```python
from build123d import *

# Parameters (mm, degrees)
EXTRUDE_1_DEPTH      = 0.4
EXTRUDE_2_DEPTH      = 0.6
EXTRUDE_3_DEPTH      = 1.3
EXTRUDE_4_DEPTH      = 1.19
FILLET_1_R           = 0.1
FILLET_2_R           = 0.1
FILLET_3_R           = 0.2
EXTRUDE_5_DEPTH      = 3.5
EXTRUDE_5_DEPTH_BACK = 3.5
EXTRUDE_5_START      = -8.2
SKETCH_3_W           = 10
SKETCH_3_H           = 10
CUT_EXTRUDE_1_DEPTH  = 0.01


with BuildPart() as part:
    # 草图1 → 凸台-拉伸1 (new body)
    with BuildSketch(Plane(origin=(0, 0, 0), x_dir=(1, 0, 0), z_dir=(0, 1, 0))):
        with BuildLine():
            Line((7.3, -8.2), (-7.3, -8.2))
            ThreePointArc((-7.3, -8.2), (-8.007106781, -7.907106781), (-8.3, -7.2))
            Line((-8.3, -7.2), (-8.3, 7.2))
            ThreePointArc((-8.3, 7.2), (-8.007106781, 7.907106781), (-7.3, 8.2))
            Line((-7.3, 8.2), (7.3, 8.2))
            ThreePointArc((7.3, 8.2), (8.007106781, 7.907106781), (8.3, 7.2))
            Line((8.3, 7.2), (8.3, -7.2))
            ThreePointArc((8.3, -7.2), (8.007106781, -7.907106781), (7.3, -8.2))
        make_face()
        with BuildLine():
            Line((7.75, -4.202947793), (7.75, 4.3))
            ThreePointArc((7.75, 4.3), (6.798097039, 6.598097039), (4.5, 7.55))
            ThreePointArc((4.5, 7.55), (4.287867966, 7.637867966), (4.2, 7.85))
            Line((4.2, 7.85), (-4.3, 7.85))
            ThreePointArc((-4.3, 7.85), (-4.387867966, 7.637867966), (-4.6, 7.55))
            ThreePointArc((-4.6, 7.55), (-6.898097039, 6.598097039), (-7.85, 4.3))
            Line((-7.85, 4.3), (-7.85, -4.2))
            ThreePointArc((-7.85, -4.2), (-6.898094676, -6.498099402), (-4.599993316, -7.45))
            ThreePointArc((-4.599993316, -7.45), (-4.387860883, -7.537867748), (-4.299992699, -7.75))
            Line((-4.299992699, -7.75), (4.200007301, -7.75))
            ThreePointArc((4.200007301, -7.75), (4.288905774, -7.539775891), (4.499993425, -7.452947793))
            ThreePointArc((4.499993425, -7.452947793), (6.798094714, -6.501047157), (7.75, -4.202947793))
        make_face(mode=Mode.SUBTRACT)
    extrude(amount=EXTRUDE_1_DEPTH)

    # 草图1<3> → 凸台-拉伸2 (add)
    with BuildSketch(Plane(origin=(0, 0, 0), x_dir=(1, 0, 0), z_dir=(0, 1, 0))):
        with BuildLine():
            Line((7.75, -4.202947793), (7.75, 4.3))
            ThreePointArc((7.75, 4.3), (6.798097039, 6.598097039), (4.5, 7.55))
            ThreePointArc((4.5, 7.55), (4.287867966, 7.637867966), (4.2, 7.85))
            Line((4.2, 7.85), (-4.3, 7.85))
            ThreePointArc((-4.3, 7.85), (-4.387867966, 7.637867966), (-4.6, 7.55))
            ThreePointArc((-4.6, 7.55), (-6.898097039, 6.598097039), (-7.85, 4.3))
            Line((-7.85, 4.3), (-7.85, -4.2))
            ThreePointArc((-7.85, -4.2), (-6.898094676, -6.498099402), (-4.599993316, -7.45))
            ThreePointArc((-4.599993316, -7.45), (-4.387860883, -7.537867748), (-4.299992699, -7.75))
            Line((-4.299992699, -7.75), (4.200007301, -7.75))
            ThreePointArc((4.200007301, -7.75), (4.288905774, -7.539775891), (4.499993425, -7.452947793))
            ThreePointArc((4.499993425, -7.452947793), (6.798094714, -6.501047157), (7.75, -4.202947793))
        make_face()
        with BuildLine():
            Line((5.15, -6.75), (-5.15, -6.75))
            ThreePointArc((-5.15, -6.75), (-6.564213562, -6.164213562), (-7.15, -4.75))
            Line((-7.15, -4.75), (-7.15, 4.75))
            ThreePointArc((-7.15, 4.75), (-6.564213562, 6.164213562), (-5.15, 6.75))
            Line((-5.15, 6.75), (5.15, 6.75))
            ThreePointArc((5.15, 6.75), (6.564213562, 6.164213562), (7.15, 4.75))
            Line((7.15, 4.75), (7.15, -4.75))
            ThreePointArc((7.15, -4.75), (6.564213562, -6.164213562), (5.15, -6.75))
        make_face(mode=Mode.SUBTRACT)
    extrude(amount=EXTRUDE_2_DEPTH)

    # 草图1<4> → 凸台-拉伸3 (add)
    with BuildSketch(Plane(origin=(0, 0, 0), x_dir=(1, 0, 0), z_dir=(0, 1, 0))):
        with BuildLine():
            Line((5.15, -6.75), (-5.15, -6.75))
            ThreePointArc((-5.15, -6.75), (-6.564213562, -6.164213562), (-7.15, -4.75))
            Line((-7.15, -4.75), (-7.15, 4.75))
            ThreePointArc((-7.15, 4.75), (-6.564213562, 6.164213562), (-5.15, 6.75))
            Line((-5.15, 6.75), (5.15, 6.75))
            ThreePointArc((5.15, 6.75), (6.564213562, 6.164213562), (7.15, 4.75))
            Line((7.15, 4.75), (7.15, -4.75))
            ThreePointArc((7.15, -4.75), (6.564213562, -6.164213562), (5.15, -6.75))
        make_face()
        with BuildLine():
            Line((5.5, -5.5), (-5.5, -5.5))
            ThreePointArc((-5.5, -5.5), (-5.782842712, -5.382842712), (-5.9, -5.1))
            Line((-5.9, -5.1), (-5.9, 5.1))
            ThreePointArc((-5.9, 5.1), (-5.782842712, 5.382842712), (-5.5, 5.5))
            Line((-5.5, 5.5), (5.5, 5.5))
            ThreePointArc((5.5, 5.5), (5.782842712, 5.382842712), (5.9, 5.1))
            Line((5.9, 5.1), (5.9, -5.1))
            ThreePointArc((5.9, -5.1), (5.782842712, -5.382842712), (5.5, -5.5))
        make_face(mode=Mode.SUBTRACT)
    extrude(amount=EXTRUDE_3_DEPTH)

    # 草图1<5> → 凸台-拉伸4 (add)
    with BuildSketch(Plane(origin=(0, 0, 0), x_dir=(1, 0, 0), z_dir=(0, 1, 0))):
        with BuildLine():
            Line((-5.9, -5.1), (-5.9, 5.1))
            ThreePointArc((-5.9, 5.1), (-5.782842712, 5.382842712), (-5.5, 5.5))
            Line((-5.5, 5.5), (5.5, 5.5))
            ThreePointArc((5.5, 5.5), (5.782842712, 5.382842712), (5.9, 5.1))
            Line((5.9, 5.1), (5.9, -5.1))
            ThreePointArc((5.9, -5.1), (5.782842712, -5.382842712), (5.5, -5.5))
            Line((5.5, -5.5), (-5.5, -5.5))
            ThreePointArc((-5.5, -5.5), (-5.782842712, -5.382842712), (-5.9, -5.1))
        make_face()
    extrude(amount=EXTRUDE_4_DEPTH)

    # 圆角1
    fillet_1_edges = [part.edges().sort_by_distance(p)[0] for p in [
        (-6.898094676, 0.6, 6.498099402),
        (-0.049992699, 0.6, 7.75),
        (4.288905774, 0.6, 7.539775891),
        (-4.387867966, 0.6, -7.637867966),
        (-7.85, 0.6, -0.05),
        (-4.387860883, 0.6, 7.537867748),
        (6.798094714, 0.6, 6.501047157),
        (7.75, 0.6, -0.048526103),
        (6.798097039, 0.6, -6.598097039),
        (4.287867966, 0.6, -7.637867966),
        (-0.05, 0.6, -7.85),
        (-6.898097039, 0.6, -6.598097039),
    ]]
    fillet(fillet_1_edges, radius=FILLET_1_R)

    # 圆角2
    fillet_2_edges = [part.edges().sort_by_distance(p)[0] for p in [
        (-6.564213562, 0.6, -6.164213562),
        (0, 0.6, -6.75),
        (6.564213562, 0.6, -6.164213562),
        (7.15, 0.6, 0),
        (6.564213562, 0.6, 6.164213562),
        (0, 0.6, 6.75),
        (-6.564213562, 0.6, 6.164213562),
        (-7.15, 0.6, 0),
    ]]
    fillet(fillet_2_edges, radius=FILLET_2_R)

    # 圆角3
    fillet_3_edges = [part.edges().sort_by_distance(p)[0] for p in [
        (-7.15, 1.3, 0),
        (-6.564213562, 1.3, 6.164213562),
        (0, 1.3, 6.75),
        (0, 1.3, -6.75),
        (-6.564213562, 1.3, -6.164213562),
        (6.564213562, 1.3, 6.164213562),
        (7.15, 1.3, 0),
        (6.564213562, 1.3, -6.164213562),
    ]]
    fillet(fillet_3_edges, radius=FILLET_3_R)

    # 草图2 → 凸台-拉伸5 (add, two sides: drawn at the far end of the back side and taken through both)
    with BuildSketch(Plane.XY.offset(8.2).offset(EXTRUDE_5_START - EXTRUDE_5_DEPTH_BACK)):
        with BuildLine():
            Line((8.3, 0.3), (9.365071607, 0.300002674))
            add(Edge.make_bspline(
                [(9.365071607, 0.300002674), (9.466251692, 0.300426751), (9.659413087, 0.300043909), (10.004363297, 0.297823417), (10.333713629, 0.295164588), (10.471404473, 0.294160487), (10.550486094, 0.293991669)],
                knots=[0.000465859, 0.000465859, 0.000465859, 0.000465859, 0.099748113, 0.199030367, 0.298312622, 0.397594876, 0.397594876, 0.397594876, 0.397594876], degree=3))
            ThreePointArc((10.550486094, 0.293991669), (11.467930406, -0.087748238), (11.847710954, -1.006005369))
            Line((11.847710954, -1.006005369), (11.847710954, -12.506005369))
            ThreePointArc((11.847710954, -12.506005369), (11.701264344, -12.85955876), (11.347710954, -13.006005369))
            Line((11.347710954, -13.006005369), (7.613209707, -13.006005369))
            Line((7.613209707, -13.006005369), (7.613209707, -12.806005369))
            Line((7.613209707, -12.806005369), (11.347710954, -12.806005369))
            ThreePointArc((11.347710954, -12.806005369), (11.559842988, -12.718137403), (11.647710954, -12.506005369))
            Line((11.647710954, -12.506005369), (11.647710954, -1.006005369))
            ThreePointArc((11.647710954, -1.006005369), (11.326358183, -0.229018566), (10.550059149, 0.093992125))
            add(Edge.make_bspline(
                [(10.550059149, 0.093992125), (10.470549094, 0.094161857), (10.331716757, 0.095173419), (10.002362016, 0.097833701), (9.657479111, 0.100049329), (9.465720155, 0.100426879), (9.365071614, 0.1000009)],
                knots=[0.000156882, 0.000156882, 0.000156882, 0.000156882, 0.099516381, 0.198875879, 0.298235377, 0.397594876, 0.397594876, 0.397594876, 0.397594876], degree=3))
            Line((9.365071614, 0.1000009), (8.3, 0.1))
            Line((8.3, 0.1), (8.3, 0.3))
        make_face()
    extrude(amount=EXTRUDE_5_DEPTH + EXTRUDE_5_DEPTH_BACK)

    # 草图3 → 切除-拉伸1 (cut)
    with BuildSketch(Plane(origin=(0, 1.19, 0), x_dir=(1, 0, 0), z_dir=(0, 1, 0))):
        with Locations((-0.4, 0)):
            Rectangle(SKETCH_3_W, SKETCH_3_H)
    extrude(amount=-CUT_EXTRUDE_1_DEPTH, mode=Mode.SUBTRACT)


solid = part.part
```
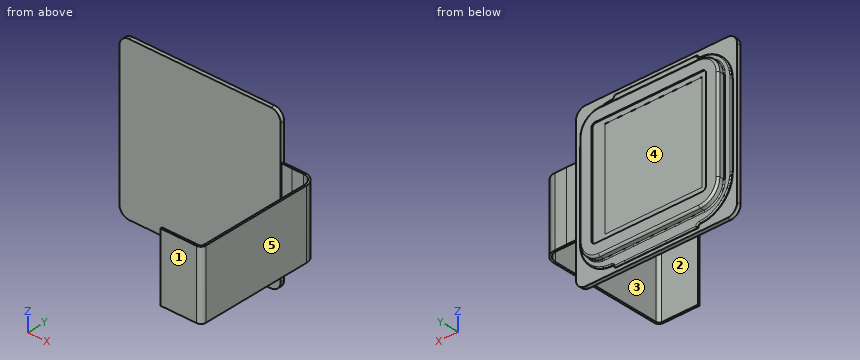
The model under review builds one solid part; all positions refer to its coordinate system, in mm. Face numbers are marked on the shaded views. A direction names the side the tool comes from. Round coordinates to 2 decimals unless told otherwise and drop trailing zeros. Order: outer loops, then holes, each group sorted by start corner. A loop starts at its lowest first (then second) coordinate and runs counter-clockwise, first axis right, second up. Notation, with made-up numbers: M 2,35 L 17,35 A27 cw 17,69 Z; hole C 20,-20 d9. An arc over 180 degrees is marked long. Use a Markdown table: item, result.
1) Wall thickness on line 1 along Y through (x, z) = (4.5, -5.25); line 2 along X through (y, z) = (-5.5, 1.75); line 3 along Y through (x, z) = (-7.5, -6.75): over which ranges is each line inside the solid? List them lowest first. Write a range as [from, to].
Report:
| item | result |
|---|---|
| line 1 | [0, 1.19] |
| line 2 | [11.65, 11.85] |
| line 3 | [0, 0.4] |
2) Consider section C-C (y = -0.75). Write out the cut boundary in (x, z), then the cut area to 3 significant figures.
Report:
| item | result |
|---|---|
| outline | M 11.62,-3.5 L 11.82,-3.5 L 11.82,3.5 L 11.62,3.5 Z |
| area | 1.43 mm^2 |
3) Draft analysis for pull direction Y (two halves, no side actions). For the marked faces 3, 4 and 5, state which applies: released by +Y, released by -Y, zero draft, split by the parting line, or undercut.
Report:
| item | result |
|---|---|
| face 3 | undercut |
| face 4 | released by +Y |
| face 5 | zero draft |
4) Insertion check: pin 1 (1.9 mm diameter, centred on x = 9.5, z = 1, fed in from +Y); pin 2 (1.5 mm diameter, centred on x = 9, y = -10, fed in from -Z); pin 3 (2 mm diameter, centred on y = -11.5, z = 0, fed in from -X); pin 4 (4.5 mm diameter, centred on x = 9.5, y = -6, fed in from +Z). Each pin has a flat end and moves straight along its axis. Give the tip position at first contact, or say it passes through.
Report:
| item | result |
|---|---|
| pin 1 | y = 0.3 |
| pin 2 | through |
| pin 3 | x = 11.65 |
| pin 4 | z = 3.5 |
5) Tool access review of the marked faces 1 and 2: name each direction out of +Z, -Z, +X, -X, +Y, -Y from which nothing blocks a thin tool from reaching the whole face with its end or side.
Report:
| item | result |
|---|---|
| face 1 | +Z, -Z, +X, -X, -Y |
| face 2 | +Z, -Z, -X |
6) Consider section B-B (y = -3.5). Write out the cut boundary in (x, z).
Report:
| item | result |
|---|---|
| outline | M 11.65,-3.5 L 11.85,-3.5 L 11.85,3.5 L 11.65,3.5 Z |
